Input: part model. Units: mm. Frame: model coordinates. A direction names the side the tool comes from. Coordinates: 2 decimals unless noted, no trailing zeros. Write each loop counter-clockwise with the first axis right and the second up, starting at its lowest first coordinate (ties: lowest second). Pieces come first, ordered by that corner, then holes. Notation, with made-up numbers: (40, -13.5) - (95, -13.5) arc R28 ccw to (95, 19.5) - close; hole circle Ø6 at (-20.5, 72.25). An arc over 180 degrees is marked (long way). Put each result on its own line as item: value. Start each with the question number.
1. Access query for faces 5 (the flat face through (2, 30, 10)), 6 (the cylindrical face through (7.715, 35.699, 10.14)), 7 (the flat face through (5, 21, 8)). Directions: +Z, -Z, +X, -X, +Y, -Y. A direction counts if a zero-diameter tool reaches every point of the face in a straight line with its end or side. Return the directions, or none.
2. Cut plane D-D, the plane z = 11.5. Return loops of the section in (x, y).
3. Line query: line 1 (Z direction, x = 1.8, y = 7.5); line 2 (Z direction, x = 5.6, y = 7.5); line 3 (Y direction, x = 5.5, z = 6.75). Output: solid intervals per line, ascending.
4. Cut plane A-A, the plane y = 22.5. Return loops of the section in (x, z).
5. Cut plane C-C, the plane x = 3.5. Return loops of the section in (y, z), and give its area (3 significant figures).
6. Pull-direction query (Z, two-part tool) for faces 1 (the flat face through (4, 18, 0)), 2 (the cylindrical face through (6.52, 21.58, 5.85)), 3 (the flat face through (5, 6, 8)), 4 (the flat face through (4.5, 33, 10)); classes: released by +Z, released by -Z, zero draft, split by the parting line, or undercut.
7. Cut plane B-B, the plane z = 17.75. Return loops of the section in (x, y).
8. Pin query (flat end, axial travel): pin 1 (4 mm diameter, centred on y = 6.5, z = 9.5, fed in from +X); pin 2 (2.5 mm diameter, centred on y = 7.5, z = 10, fed in from -X); pin 3 (5.5 mm diameter, centred on y = 33, z = 13, fed in from -X); pin 4 (1.3 mm diameter, centred on x = 3, z = 8, fed in from +Y). Return the tip coordinate at first contact, or that it passes through.
from build123d import *

# Parameters (mm, degrees)
F1_DEPTH = 20
F2_R     = 2
F3_DEPTH = 8.001
F4_R     = 1
F5_R     = 4.25
F6_DEPTH = 3


with BuildPart() as f1:
    # F0 (on Top) → F1 (new body)
    with BuildSketch(Plane.XY):
        Polygon((8, 0), (8, 36), (4.5, 36), (4.5, 30), (0, 30), (0, 0), align=None)
    extrude(amount=F1_DEPTH)

    # F2 (on face) → F3 (cut, through all)
    with BuildSketch(Plane(origin=(0, 0, 0), x_dir=(0, -1, 0), z_dir=(-1, 0, 0))):
        with Locations((-7.5, 10)):
            Circle(F2_R)
        with Locations((-22.5, 10)):
            Circle(F2_R)
    extrude(amount=-F3_DEPTH, mode=Mode.SUBTRACT)

    # F4
    f4_edges = [f1.edges().sort_by_distance(p)[0] for p in [
        (4.5, 36, 10),
        (8, 36, 10),
    ]]
    fillet(f4_edges, radius=F4_R)

    # F5 (on face) → F6 (cut)
    with BuildSketch(Plane.YZ.offset(8)):
        with Locations((22.5, 10)):
            Circle(F5_R)
        with Locations((7.5, 10)):
            Circle(F5_R)
    extrude(amount=-F6_DEPTH, mode=Mode.SUBTRACT)


solid = f1.part
Report:
1. face 5: +Z, -Z, -X, +Y
1. face 6: +Z, -Z, +X, +Y
1. face 7: +X
2. outline: (0, 0) - (8, 0) - (8, 3.52) - (5, 3.52) - (5, 6.18) - (0, 6.18) - close; (0, 8.82) - (5, 8.82) - (5, 11.48) - (8, 11.48) - (8, 18.52) - (5, 18.52) - (5, 21.18) - (0, 21.18) - close; (0, 23.82) - (5, 23.82) - (5, 26.48) - (8, 26.48) - (8, 35) arc R1 ccw to (7, 36) - (5.5, 36) arc R1 ccw to (4.5, 35) - (4.5, 30) - (0, 30) - close
3. line 1: z = 0 to 8, 12 to 20
3. line 2: z = 0 to 5.75, 14.25 to 20
3. line 3: y = 0 to 4.76, 10.24 to 19.76, 25.24 to 36
4. outline: (0, 0) - (8, 0) - (8, 5.75) - (5, 5.75) - (5, 8) - (0, 8) - close; (0, 12) - (5, 12) - (5, 14.25) - (8, 14.25) - (8, 20) - (0, 20) - close
5. outline: (0, 0) - (30, 0) - (30, 20) - (0, 20) - close; hole circle Ø4 at (7.5, 10); hole circle Ø4 at (22.5, 10)
5. area: 575 mm^2
6. face 1: released by -Z
6. face 2: undercut
6. face 3: undercut
6. face 4: zero draft
7. outline: (0, 0) - (8, 0) - (8, 35) arc R1 ccw to (7, 36) - (5.5, 36) arc R1 ccw to (4.5, 35) - (4.5, 30) - (0, 30) - close
8. pin 1: stops at x = 5
8. pin 2: passes through
8. pin 3: stops at x = 4.5
8. pin 4: stops at y = 30
